Can you work these out from the model? Positions are in its coordinate system, mm. A direction names the side the tool comes from. Round coordinates to 2 decimals unless told otherwise and drop trailing zeros. Loops run counter-clockwise (first coordinate to the right, second up) from the corner with the lowest first, then second, coordinate; pieces in that order, holes last. Notation, with made-up numbers: (4.5, 2) -> (28.5, 2) arc R12 cw to (28.5, 8) -> close; hole circle Ø5 at (-20.5, -6). An arc over 180 degrees is marked (long way). Use a Markdown table: item, result.
from build123d import *

# Parameters (mm, degrees)
SKETCH2_W           = 114.3
SKETCH2_H           = 38.1
BOSS_EXTRUDE2_DEPTH = 5.334
SKETCH3_W           = 16.256
SKETCH3_H           = 38.1
CUT_EXTRUDE3_DEPTH  = 61.477074632
CAVITY1_START       = -19.05
CAVITY1_OUTLINE_W   = 5.334
CAVITY1_OUTLINE_H   = 16.328571429
CAVITY1_DEPTH       = 5.334


# Read off the part's stored shape, not the designer's step: Cavity1
with BuildPart() as part:
    # Sketch2 → Boss-Extrude2 (new body)
    with BuildSketch(Plane(origin=(0, 0, 0), x_dir=(0, 0, -1), z_dir=(1, 0, 0))):
        Rectangle(SKETCH2_W, SKETCH2_H)
    extrude(amount=BOSS_EXTRUDE2_DEPTH)

    # Sketch3 → Cut-Extrude3 (cut, through all)
    with BuildSketch(Plane(origin=(5.334, 0, 0), x_dir=(0, 0, -1), z_dir=(1, 0, 0))):
        with Locations((49.022, 0)):
            Rectangle(SKETCH3_W, SKETCH3_H)
    extrude(amount=-CUT_EXTRUDE3_DEPTH, mode=Mode.SUBTRACT)

    # Cavity1 outline → Cavity1 (cut)
    with BuildSketch(Plane(origin=(0, 0, 0), x_dir=(1, 0, 0), z_dir=(0, 1, 0)).offset(CAVITY1_START)):
        with Locations((2.667, 32.729714286)):
            Rectangle(CAVITY1_OUTLINE_W, CAVITY1_OUTLINE_H)
        with Locations((2.667, 0.072571428)):
            Rectangle(CAVITY1_OUTLINE_W, CAVITY1_OUTLINE_H)
        with Locations((2.667, -32.584571428)):
            Rectangle(CAVITY1_OUTLINE_W, CAVITY1_OUTLINE_H)
    extrude(amount=CAVITY1_DEPTH, mode=Mode.SUBTRACT)


solid = part.part
1. I need wall thicknesses on line 1 (Z direction, x = 4.45, y = -14.5); line 2 (Y direction, x = 4.25, z = -25). Which ranges of each line are inside material? Lowest first, please.
Answer sheet:
| item | result |
|---|---|
| line 1 | z = -24.57 to -8.24, 8.09 to 24.42, 40.75 to 57.15 |
| line 2 | y = -13.72 to 19.05 |
2. I want a section at A-A (x = 2.3). Please give me the cut outline in (y, z), plus the area to 3 significant figures.
Answer sheet:
| item | result |
|---|---|
| outline | (-19.05, -24.57) -> (-13.72, -24.57) -> (-13.72, -40.89) -> (19.05, -40.89) -> (19.05, 57.15) -> (-19.05, 57.15) -> (-19.05, 40.75) -> (-13.72, 40.75) -> (-13.72, 24.42) -> (-19.05, 24.42) -> (-19.05, 8.09) -> (-13.72, 8.09) -> (-13.72, -8.24) -> (-19.05, -8.24) -> close |
| area | 3,470 mm² |
3. Which directions (+Z, -Z, +X, -X, +Y, -Y) give clear straight access to the entire face, cutting with the end or side of a thin tool? Please do faces 1 (the flat face through (3, -16, -24.565)), 2 (the flat face through (3, -13.716, 32)), 3 (the flat face through (3, 19.05, 9)).
Answer sheet:
| item | result |
|---|---|
| face 1 | -Z, +X, -X, -Y |
| face 2 | +X, -X, -Y |
| face 3 | +Z, -Z, +X, -X, +Y |
4. If we mould it in two halves opening along Z, with no side actions, what happens to faces 4 (the flat face through (3, 2, -40.894)), 5 (the flat face through (3, -16, -8.237)), 6 (the flat face through (3, -19.05, 49))? For each: +Z half, -Z half, draft (parallel to the pull), parting line (faces both ways), or undercut.
Answer sheet:
| item | result |
|---|---|
| face 4 | -Z half |
| face 5 | undercut |
| face 6 | draft |
5. Will these pins go through, and if not, where does the flat tip stop? pin 1 Ø2.5 at (x, y) = (3, -16) entering from -Z; pin 2 Ø1.6 at (x, z) = (3.5, 29.5) entering from -Y.
Answer sheet:
| item | result |
|---|---|
| pin 1 | stops at z = -24.57 |
| pin 2 | stops at y = -13.72 |
